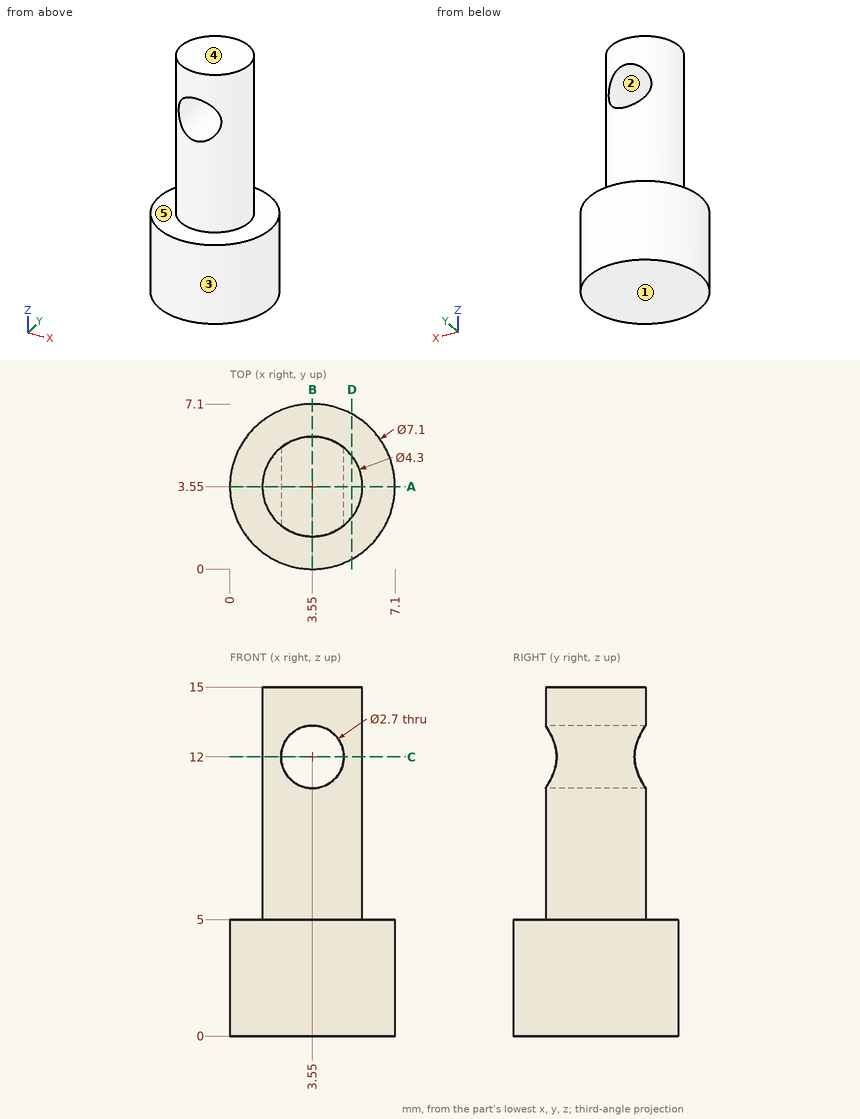
Study the drawing (mm; zero at the part's minimum x, y, z) and answer. A direction names the side the tool comes from. Coordinates: 2 decimals unless noted, no trailing zeros. Loops run counter-clockwise (first coordinate to the right, second up) from the corner with the lowest first, then second, coordinate; pieces in that order, holes last. Notation, with made-up numbers: M -31,88 L 1,88 A21 cw 1,108 Z; hole C -14.5,79 d9. An arc over 180 degrees is marked long. Answer in a Markdown table with one row per item. Add a question column.
1. A flat-ended cylindrical pin translates along its axis: P1, Ø4, axis at x = 4.5, z = 1.5, coming from the -Y side. Find the tip coordinate at first contact, or state that the pin passes through.
2. Find section D-D, the plane x = 5.25. Write down the section's boundary in (y, z), then the cut area to 3 significant figures.
3. The mould has two halves that part along Z. Classify the marked faces 1, 2 and 3: pulls with the +Z half, pulls with the -Z half, needs draft (parallel to the pull), parting line crosses it, or undercut.
4. Find section B-B, the plane x = 3.55. Write down the section's boundary in (y, z).
5. A tool of negligible diameter and unlimited length cuts with its end or side. For the marked faces 4 and 5, from which of +Z, -Z, +X, -X, +Y, -Y can it reach the whole face along a straight path? Write none if from no direction.
6. Find section C-C, the plane z = 12. Write down the section's boundary in (x, y).
7. Find section A-A, the plane y = 3.55. Write down the section's boundary in (x, z), then the cut area to 3 significant figures.
8. Consider L1, parallel to Z at x = 3.55, y = 2.5; L2, parallel to Z at x = 0.5, y = 4.5; L3, parallel to Z at x = 4.25, y = 1.75. Determine where each line is inside the solid, lowest interval first.
Reported:
| question | item | result |
|---|---|---|
| 1 | P1 | stops at y = 0 |
| 2 | outline | M 0.43,0 L 6.67,0 L 6.67,5 L 4.87,5 L 4.87,15 L 2.23,15 L 2.23,5 L 0.43,5 Z |
| 2 | area | 57.5 mm^2 |
| 3 | face 1 | pulls with the -Z half |
| 3 | face 2 | undercut |
| 3 | face 3 | needs draft |
| 4 | outline | M 0,0 L 7.1,0 L 7.1,5 L 5.7,5 L 5.7,10.65 L 1.4,10.65 L 1.4,5 L 0,5 Z; M 1.4,13.35 L 5.7,13.35 L 5.7,15 L 1.4,15 Z |
| 5 | face 4 | +Z, +X, -X, +Y, -Y |
| 5 | face 5 | +Z |
| 6 | outline | M 2.2,1.88 L 2.2,5.22 A2.15 ccw Z; M 4.9,1.88 A2.15 ccw 4.9,5.22 Z |
| 7 | outline | M 0,0 L 7.1,0 L 7.1,5 L 5.7,5 L 5.7,15 L 1.4,15 L 1.4,5 L 0,5 Z; hole C 3.55,12 d2.7 |
| 7 | area | 72.8 mm^2 |
| 8 | L1 | z = 0 to 10.65, 13.35 to 15 |
| 8 | L2 | z = 0 to 5 |
| 8 | L3 | z = 0 to 10.85, 13.15 to 15 |
